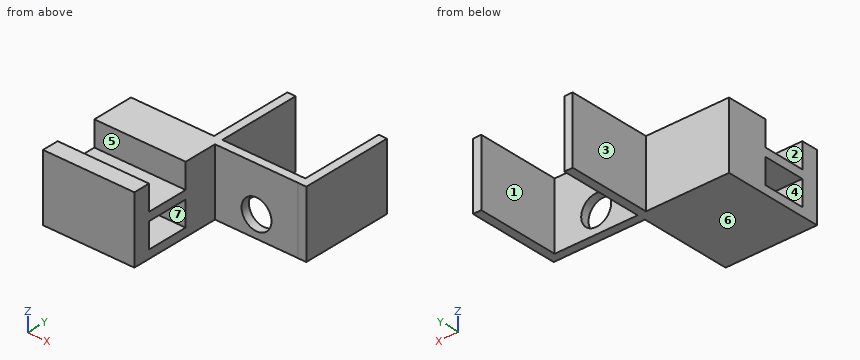
Autodesk Inventor part; units mm, degrees
ref_plane "YZ Plane" through (0, 0, 0) normal (1, 0, 0) x (0, 1, 0)
ref_plane "XZ Plane" through (0, 0, 0) normal (0, 1, 0) x (-1, 0, 0)
ref_plane "XY Plane" through (0, 0, 0) normal (0, 0, 1) x (1, 0, 0)
sketch "Sketch1" plane through (0, 0, 0) normal (0, 0, 1) x (1, 0, 0)
  line L0 (-25, 25) -> (25, 25)
  line L1 (25, 25) -> (25, -30)
  line L2 (30, -25) -> (-30, -25)
  line L3 (-25, -30) -> (-25, 80)
  line L4 (-25, 25) -> (25, -25) construction
  line L5 (25, 25) -> (-25, -25) construction
  line L6 (25, 25) -> (-51, 25)
  line L7 (25, 80) -> (25, 25)
  line L8 (-51, 25) -> (-75, 25)
  line L9 (-75, 25) -> (-75, -25)
  line L10 (-75, -25) -> (-30, -25)
  line L11 (30, 30) -> (-30, 30)
  line L12 (-30, 30) -> (-30, -30)
  line L13 (-30, -30) -> (30, -30)
  line L14 (30, -30) -> (30, 30)
  line L15 (30, 25) -> (30, 80)
  line L16 (-30, 80) -> (-30, 25)
  line L17 (-80, -30) -> (-80, 30)
  line L18 (-80, 30) -> (-30, 30)
  line L19 (-30, -30) -> (-80, -30)
  line L20 (-30, 80) -> (30, 80)
  line L21 (24.924, 24.924) -> (30, 25)
  point P0 (0, 0)
  point P1 (25, 30)
  point P2 (-30, 25)
  point P3 (-25, 30)
  point P4 (25, 24.9251)
  dimension "d4" = 5
  dimension "d7" = 50
  dimension "d8" = 0
  dimension "d9" = 5
  dimension "d12" = 55
  dimension "d13" = 60
  dimension "d14" = 105
  dimension "d15" = 50
  dimension "d18" = 110
  dimension "d19" = 3.5355
  dimension "d20" = 38.8909
  dimension "d21" = 81
extrude "Extrusion1" add sketch "Sketch1" along normal blind 40 contours L3 L11 L7 L0 | L6 L12 L11 L3 | L3 L2 L12 L6 | L7 L11 L14 L21 L1 | L3 L13 L12 L2 | L11 L16 L20 L3 | L12 L10 L9 L8 L6 | L6 L8 L9 L10 L12 L19 L17 L18 | L7 L20 L15 L11
sketch "Sketch2" plane through (-25, 25, 0) normal (0, -1, 0) x (1, 0, 0)
  circle A0 centre (25, 13) radius 9
  line L0 (0, 0) -> (50, 0)
  point P0 (25, 0)
  dimension "d24" = 18
  dimension "d25" = 13
extrude "Extrusion2" cut sketch "Sketch2" against normal blind 40
sketch "Sketch3" plane through (-25, -30, 0) normal (1, 0, 0) x (0, 0, -1)
  line L0 (0, 0) -> (-40, 0)
  line L1 (0, 55) -> (-40, 55)
  line L2 (0, 0) -> (-5, 0)
  line L3 (-5, 0) -> (-5, 55)
  line L4 (-5, 55) -> (0, 55)
  line L5 (0, 55) -> (0, 0)
  line L6 (-5, 0) -> (-20, 0)
  line L7 (-20, 0) -> (-20, 55)
  line L8 (-20, 55) -> (-5, 55)
  line L9 (-5, 55) -> (-5, 0)
  line L10 (-20, 0) -> (-25, 0)
  line L11 (-25, 0) -> (-25, 55)
  line L12 (-25, 55) -> (-20, 55)
  line L13 (-20, 55) -> (-20, 0)
  line L14 (-25, 0) -> (-40, 0)
  line L15 (-40, 0) -> (-40, 55)
  line L16 (-40, 55) -> (-25, 55)
  line L17 (-25, 55) -> (-25, 0)
  line L18 (-40, 0) -> (0, 0)
  line L19 (0, 0) -> (0, 10)
  line L20 (0, 10) -> (-40, 10)
  line L21 (-40, 10) -> (-40, 0)
  line L22 (-40, 55) -> (-20, 55)
  line L23 (-20, 55) -> (-20, 37.9712)
  line L24 (-20, 37.9712) -> (-40, 37.9712)
  line L25 (-40, 37.9712) -> (-40, 55)
  line L26 (-40, 55) -> (-5, 55)
  line L27 (-5, 55) -> (-5, 35)
  line L28 (-5, 35) -> (-40, 35)
  line L29 (-40, 35) -> (-40, 55)
  point P0 (0, 30)
  point P1 (-20, 10)
  point P2 (-5, 10)
  point P3 (-25, 10)
  point P4 (-20, 35)
  point P5 (-25, 35)
  dimension "d28" = 5
  dimension "d29" = 15
  dimension "d30" = 5
  dimension "d33" = 10
  dimension "d34" = 20
  dimension "d35" = 20
extrude "Extrusion3" cut sketch "Sketch3" against normal through all contours L20 L7 L28 L3 | L20 L15 L28 L11
Source: CAD feature listing. Evaluate the final solid. Frame: model axes, mm. Face numbers are marked on the shaded views. A direction names the side the tool comes from. Coordinates: 2 decimals unless noted, no trailing zeros. Loops run counter-clockwise (first coordinate to the right, second up) from the corner with the lowest first, then second, coordinate; pieces in that order, holes last. Notation, with made-up numbers: M 15,0.5 L 62,0.5 A23 ccw 62,11.5 Z; hole C 57.5,47 d10. An arc over 180 degrees is marked long. Use a Markdown table: item, result. Add a question column.
Q1. Section query D-D, the plane z = 35.5. Return loops of the section in (x, y), and give its area (3 significant figures).
Q2. Section query B-B, the plane x = 0. Return loops of the section in (y, z).
Q3. Draft query along Z for the marked faces 4, 5, 6 and 7. Return one class per face: pulls with the +Z half, pulls with the -Z half, needs draft (parallel to the pull), parting line crosses it, or undercut.
Q4. First-contact query: pin 1 (7.5 mm diameter, centred on x = -46.5, z = 13, fed in from +Y); pin 2 (8 mm diameter, centred on y = 67.5, z = 9.5, fed in from -X); pin 3 (12.5 mm diameter, centred on x = -53.5, y = -11.5, fed in from +Z). Flat tips, straight axial feed; report the tip coordinate or a pass-through.
Q5. Access query for the marked faces 1, 2 and 3. Directions: +Z, -Z, +X, -X, +Y, -Y. A direction counts if a zero-diameter tool reaches every point of the face in a straight line with its end or side. Return the directions, or none.
Q6. Section query C-C, the plane y = 56.5. Return loops of the section in (x, z), and give its area (3 significant figures).
Q7. Material intervals for L1, parallel to X at y = 50, z = 32; L2, parallel to Z at x = 0, y = 28.6; L3, parallel to Y at x = -68, z = 35, sorted ascending.
Q8. Section query A-A, the plane z = 13. Return loops of the section in (x, y).
Result:
| question | item | result |
|---|---|---|
| 1 | outline | M -80,-30 L -25,-30 L -25,-20 L -80,-20 Z; M -80,5 L -25,5 L -25,25 L 25,25 L 25,24.93 L 30,25 L 30,80 L 25,80 L 25,30 L -25,30 L -25,80 L -30,80 L -30,30 L -80,30 Z |
| 1 | area | 2,700 mm2 |
| 2 | outline | M 25,0 L 30,0 L 30,4 L 25,4 Z; M 25,22 L 30,22 L 30,40 L 25,40 Z |
| 3 | face 4 | undercut |
| 3 | face 5 | needs draft |
| 3 | face 6 | pulls with the -Z half |
| 3 | face 7 | undercut |
| 4 | pin 1 | stops at y = 30 |
| 4 | pin 2 | stops at x = -30 |
| 4 | pin 3 | stops at z = 25 |
| 5 | face 1 | +Z, -Z, +Y |
| 5 | face 2 | +Z, +X, -X |
| 5 | face 3 | +Z, -Z, -X, +Y |
| 6 | outline | M -30,0 L -25,0 L -25,40 L -30,40 Z; M 25,0 L 30,0 L 30,40 L 25,40 Z |
| 6 | area | 400 mm2 |
| 7 | L1 | x = -30 to -25, 25 to 30 |
| 7 | L2 | z = 0 to 4, 22 to 40 |
| 7 | L3 | y = -30 to -20, 5 to 30 |
| 8 | outline | M -80,-30 L -25,-30 L -25,-20 L -80,-20 Z; M -80,5 L -25,5 L -25,25 L -9,25 L -9,30 L -25,30 L -25,80 L -30,80 L -30,30 L -80,30 Z; M 9,25 L 25,25 L 25,24.93 L 30,25 L 30,80 L 25,80 L 25,30 L 9,30 Z |
